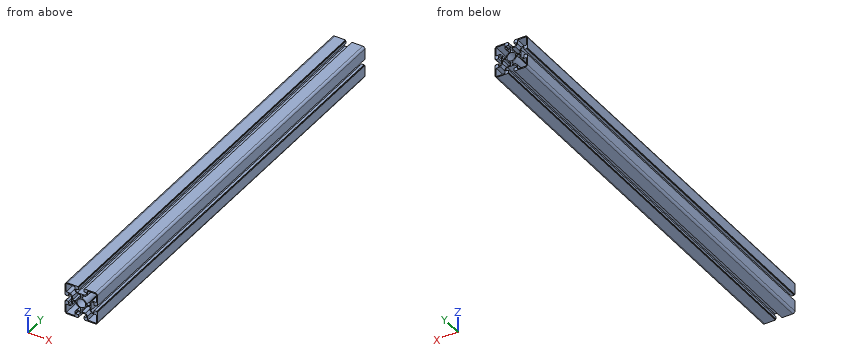
```python
from build123d import *

# Parameters (mm, degrees)
SKETCH_1_R      = 8
EXTRUDE_1_DEPTH = 800


with BuildPart() as part:
    # 草图1 → 凸台-拉伸1 (new body)
    with BuildSketch(Plane(origin=(0, 0, 0), x_dir=(1, 0, 0), z_dir=(0, 1, 0))):
        with BuildLine():
            Line((-30, 5.999999999), (-28.5, 5.999999999))
            Line((-28.5, 5.999999999), (-28.5, 4.999999999))
            Line((-28.5, 4.999999999), (-24, 4.999999999))
            Line((-24, 4.999999999), (-24, 9.999999999))
            Line((-24, 9.999999999), (-21, 9.999999999))
            Line((-21, 9.999999999), (-18, 6.999999999))
            Line((-18, 6.999999999), (-18, -7.000000001))
            Line((-18, -7.000000001), (-21, -10.000000001))
            Line((-21, -10.000000001), (-24, -10.000000001))
            Line((-24, -10.000000001), (-24, -5.000000001))
            Line((-24, -5.000000001), (-28.5, -5.000000001))
            Line((-28.5, -5.000000001), (-28.5, -6.000000001))
            Line((-28.5, -6.000000001), (-30, -6.000000001))
            Line((-30, -6.000000001), (-30, -26.000000001))
            ThreePointArc((-30, -26.000000001), (-28.828427125, -28.828427126), (-26, -30.000000001))
            Line((-26, -30.000000001), (-6, -30.000000001))
            Line((-6, -30.000000001), (-6, -28.500000001))
            Line((-6, -28.500000001), (-5, -28.500000001))
            Line((-5, -28.500000001), (-5, -24.000000001))
            Line((-5, -24.000000001), (-10, -24.000000001))
            Line((-10, -24.000000001), (-10, -21.000000001))
            Line((-10, -21.000000001), (-7, -18.000000001))
            Line((-7, -18.000000001), (7, -18.000000001))
            Line((7, -18.000000001), (10, -21.000000001))
            Line((10, -21.000000001), (10, -24.000000001))
            Line((10, -24.000000001), (5, -24.000000001))
            Line((5, -24.000000001), (5, -28.500000001))
            Line((5, -28.500000001), (6, -28.500000001))
            Line((6, -28.500000001), (6, -30.000000001))
            Line((6, -30.000000001), (26, -30.000000001))
            ThreePointArc((26, -30.000000001), (28.828427125, -28.828427126), (30, -26.000000001))
            Line((30, -26.000000001), (30, -6.000000001))
            Line((30, -6.000000001), (28.5, -6.000000001))
            Line((28.5, -6.000000001), (28.5, -5.000000001))
            Line((28.5, -5.000000001), (24, -5.000000001))
            Line((24, -5.000000001), (24, -10.000000001))
            Line((24, -10.000000001), (21, -10.000000001))
            Line((21, -10.000000001), (18, -7.000000001))
            Line((18, -7.000000001), (18, 6.999999999))
            Line((18, 6.999999999), (21, 9.999999999))
            Line((21, 9.999999999), (24, 9.999999999))
            Line((24, 9.999999999), (24, 4.999999999))
            Line((24, 4.999999999), (28.5, 4.999999999))
            Line((28.5, 4.999999999), (28.5, 5.999999999))
            Line((28.5, 5.999999999), (30, 5.999999999))
            Line((30, 5.999999999), (30, 25.999999999))
            ThreePointArc((30, 25.999999999), (28.828427125, 28.828427124), (26, 29.999999999))
            Line((26, 29.999999999), (6, 29.999999999))
            Line((6, 29.999999999), (6, 28.499999999))
            Line((6, 28.499999999), (5, 28.499999999))
            Line((5, 28.499999999), (5, 23.999999999))
            Line((5, 23.999999999), (10, 23.999999999))
            Line((10, 23.999999999), (10, 20.999999999))
            Line((10, 20.999999999), (7, 17.999999999))
            Line((7, 17.999999999), (-7, 17.999999999))
            Line((-7, 17.999999999), (-10, 20.999999999))
            Line((-10, 20.999999999), (-10, 23.999999999))
            Line((-10, 23.999999999), (-5, 23.999999999))
            Line((-5, 23.999999999), (-5, 28.499999999))
            Line((-5, 28.499999999), (-6, 28.499999999))
            Line((-6, 28.499999999), (-6, 29.999999999))
            Line((-6, 29.999999999), (-26.000000001, 29.999999999))
            ThreePointArc((-26.000000001, 29.999999999), (-28.828427125, 28.828427123), (-30, 25.999999999))
            Line((-30, 25.999999999), (-30, 5.999999999))
        make_face()
        with Locations(Location((0, 0, 0), (0, 0, 270))):
            Circle(SKETCH_1_R, mode=Mode.SUBTRACT)
        with BuildLine():
            Line((-16, 1), (-9.949874371, 1))
            ThreePointArc((-9.949874371, 1), (-7.071067812, 7.071067811), (-1.000000001, 9.949874371))
            Line((-1.000000001, 9.949874371), (-1.000000001, 16))
            Line((-1.000000001, 16), (-7.828427125, 16))
            Line((-7.828427125, 16), (-12, 20.171572875))
            Line((-12, 20.171572875), (-12, 28))
            Line((-12, 28), (-28, 28))
            Line((-28, 28), (-28, 12))
            Line((-28, 12), (-20.171572875, 12))
            Line((-20.171572875, 12), (-16, 7.828427125))
            Line((-16, 7.828427125), (-16, 1))
        make_face(mode=Mode.SUBTRACT)
        with BuildLine():
            Line((1, 9.949874371), (1, 16))
            Line((1, 16), (7.828427125, 16))
            Line((7.828427125, 16), (12, 20.171572875))
            Line((12, 20.171572875), (12, 28))
            Line((12, 28), (28, 28))
            Line((28, 28), (28, 12.000000001))
            Line((28, 12.000000001), (20.171572875, 12.000000001))
            Line((20.171572875, 12.000000001), (16, 7.828427126))
            Line((16, 7.828427126), (16, 1.000000001))
            Line((16, 1.000000001), (9.949874371, 1.000000001))
            ThreePointArc((9.949874371, 1.000000001), (7.071067811, 7.071067812), (1, 9.949874371))
        make_face(mode=Mode.SUBTRACT)
        with BuildLine():
            Line((9.949874371, -1), (16, -1))
            Line((16, -1), (16, -7.828427125))
            Line((16, -7.828427125), (20.171572875, -12))
            Line((20.171572875, -12), (28.000000001, -12))
            Line((28.000000001, -12), (28.000000001, -28))
            Line((28.000000001, -28), (12.000000001, -28))
            Line((12.000000001, -28), (12.000000001, -20.171572875))
            Line((12.000000001, -20.171572875), (7.828427126, -16))
            Line((7.828427126, -16), (1.000000001, -16))
            Line((1.000000001, -16), (1.000000001, -9.949874371))
            ThreePointArc((1.000000001, -9.949874371), (7.071067812, -7.071067811), (9.949874371, -1))
        make_face(mode=Mode.SUBTRACT)
        with BuildLine():
            Line((-1, -9.949874371), (-1, -16.000000001))
            Line((-1, -16.000000001), (-7.828427125, -16.000000001))
            Line((-7.828427125, -16.000000001), (-12, -20.171572876))
            Line((-12, -20.171572876), (-12, -28.000000001))
            Line((-12, -28.000000001), (-28, -28.000000001))
            Line((-28, -28.000000001), (-28, -12.000000001))
            Line((-28, -12.000000001), (-20.171572875, -12.000000001))
            Line((-20.171572875, -12.000000001), (-16, -7.828427126))
            Line((-16, -7.828427126), (-16, -1.000000001))
            Line((-16, -1.000000001), (-9.949874371, -1.000000001))
            ThreePointArc((-9.949874371, -1.000000001), (-7.071067811, -7.071067812), (-1, -9.949874371))
        make_face(mode=Mode.SUBTRACT)
    extrude(amount=EXTRUDE_1_DEPTH)


solid = part.part
```
Geometry check sheet. Reference: the model listing, model coordinates, mm. Give positions to 0.01 mm unless a question says otherwise; leave off trailing zeros. Use one line per item in the form item = value.
Item 1: Scan lines: line 1 (X direction, y = 458, z = 25.5); line 2 (X direction, y = 117, z = -27); line 3 (Z direction, x = -12.5, y = 656). Record each from-to range of solid material in increasing order.
Results list:
line_1 = -30 to -28, -12 to -5, 5 to 12, 28 to 30
line_2 = -29.87 to -28, -12 to -5, 5 to 12, 28 to 29.87
line_3 = -30 to -28, -1 to 1, 28 to 30
Item 2: Depth check by flat-ended pin: pin 1 Ø1.2 at (x, y) = (-29.5, 254) entering from +Z (3 decimals); pin 2 Ø10 at (y, z) = (183.5, 0.5) entering from -X; pin 3 Ø0.8 at (x, y) = (5.5, 538.5) entering from +Z. Enter the tip coordinate at first touch or a pass-through.
Results list:
pin_1 = 28.755
pin_2 = -28.5
pin_3 = 28.5
Item 3: Sectioned sample at A-A on y = 386.5. Count the separate pieces of the cut face and the enclosed holes in it, plus the area to 3 significant figures.
Results list:
separate_pieces = 1
enclosed_holes = 5
area = 998 mm2
